```python
from build123d import *

# Parameters (mm, degrees)
CROQUIS1_W                = 220
CROQUIS1_H                = 153
SALIENTE_EXTRUIR1_DEPTH   = 3
CROQUIS2_W                = 160
CROQUIS2_H                = 94
CORTAR_EXTRUIR1_DEPTH     = 4
CROQUIS3_R                = 4.1
CORTAR_EXTRUIR2_DEPTH     = 4
CROQUIS4_R                = 5
SALIENTE_EXTRUIR2_DEPTH   = 7
CROQUIS5_R                = 1.5
CORTAR_EXTRUIR3_DEPTH     = 11
CORTAR_EXTRUIR4_DEPTH     = 3
SIMETR_A2_COPY_1_SKETCH_R = 4.1
SIMETR_A2_COPY_1_DEPTH    = 4
SIMETR_A2_COPY_2_SKETCH_R = 5
SIMETR_A2_COPY_2_DEPTH    = 7
SIMETR_A2_COPY_3_SKETCH_R = 1.5
SIMETR_A2_COPY_3_DEPTH    = 11
SIMETR_A2_COPY_4_DEPTH    = 3
SIMETR_A2_COPY_5_SKETCH_R = 5
SIMETR_A2_COPY_5_DEPTH    = 7
SIMETR_A2_COPY_6_SKETCH_R = 1.5
SIMETR_A2_COPY_6_DEPTH    = 11
SIMETR_A2_COPY_7_DEPTH    = 3


with BuildPart() as part:
    # Croquis1 → Saliente-Extruir1 (new body)
    with BuildSketch(Plane(origin=(0, 0, 0), x_dir=(1, 0, 0), z_dir=(0, 1, 0))):
        Rectangle(CROQUIS1_W, CROQUIS1_H)
    extrude(amount=SALIENTE_EXTRUIR1_DEPTH)

    # Croquis2 → Cortar-Extruir1 (cut, through all)
    with BuildSketch(Plane(origin=(0, 3, 0), x_dir=(1, 0, 0), z_dir=(0, 1, 0))):
        Rectangle(CROQUIS2_W, CROQUIS2_H)
    cortar_extruir1 = extrude(amount=-CORTAR_EXTRUIR1_DEPTH, mode=Mode.SUBTRACT)

    # Croquis3 → Cortar-Extruir2 (cut, through all)
    with BuildSketch(Plane(origin=(0, 3, 0), x_dir=(1, 0, 0), z_dir=(0, 1, 0))):
        with Locations((-100, 61.5)):
            Circle(CROQUIS3_R)
    cortar_extruir2 = extrude(amount=-CORTAR_EXTRUIR2_DEPTH, mode=Mode.SUBTRACT)

    # Croquis4 → Saliente-Extruir2 (add)
    with BuildSketch(Plane(origin=(0, 3, 0), x_dir=(1, 0, 0), z_dir=(0, 1, 0))):
        with Locations((-78.5, 57.5)):
            Circle(CROQUIS4_R)
    saliente_extruir2 = extrude(amount=SALIENTE_EXTRUIR2_DEPTH)

    # Croquis5 → Cortar-Extruir3 (cut, through all)
    with BuildSketch(Plane(origin=(0, 10, 0), x_dir=(1, 0, 0), z_dir=(0, 1, 0))):
        with Locations((-78.5, 57.5)):
            Circle(CROQUIS5_R)
    cortar_extruir3 = extrude(amount=-CORTAR_EXTRUIR3_DEPTH, mode=Mode.SUBTRACT)

    # Croquis6 → Cortar-Extruir4 (cut)
    with BuildSketch(Plane.XZ):
        Polygon((-81.675426481, -57.5), (-80.08771324, -60.25), (-76.91228676, -60.25), (-75.324573519, -57.5), (-76.91228676, -54.75), (-80.08771324, -54.75), align=None)
    cortar_extruir4 = extrude(amount=-CORTAR_EXTRUIR4_DEPTH, mode=Mode.SUBTRACT)

    # Simetría1: Cortar-Extruir2, Saliente-Extruir2, Cortar-Extruir3, Cortar-Extruir4 across plane
    add(cortar_extruir2.mirror(Plane(origin=(0, 0, 0), x_dir=(0, 0, 1), z_dir=(1, 0, 0))), mode=Mode.SUBTRACT)
    add(saliente_extruir2.mirror(Plane(origin=(0, 0, 0), x_dir=(0, 0, 1), z_dir=(1, 0, 0))))
    add(cortar_extruir3.mirror(Plane(origin=(0, 0, 0), x_dir=(0, 0, 1), z_dir=(1, 0, 0))), mode=Mode.SUBTRACT)
    add(cortar_extruir4.mirror(Plane(origin=(0, 0, 0), x_dir=(0, 0, 1), z_dir=(1, 0, 0))), mode=Mode.SUBTRACT)

    # Simetría2: Cortar-Extruir1, Cortar-Extruir2 across plane
    add(cortar_extruir1.mirror(Plane.XY), mode=Mode.SUBTRACT)
    add(cortar_extruir2.mirror(Plane.XY), mode=Mode.SUBTRACT)

    # Simetría2 copy 1 sketch → Simetría2 copy 1 (cut, through all)
    with BuildSketch(Plane(origin=(0, 3, 0), x_dir=(-1, 0, 0), z_dir=(0, 1, 0))):
        with Locations((-100, 61.5)):
            Circle(SIMETR_A2_COPY_1_SKETCH_R)
    extrude(amount=-SIMETR_A2_COPY_1_DEPTH, mode=Mode.SUBTRACT)

    # Simetría2 copy 2 sketch → Simetría2 copy 2 (add)
    with BuildSketch(Plane(origin=(0, 3, 0), x_dir=(-1, 0, 0), z_dir=(0, 1, 0))):
        with Locations((-78.5, 57.5)):
            Circle(SIMETR_A2_COPY_2_SKETCH_R)
    extrude(amount=SIMETR_A2_COPY_2_DEPTH)

    # Simetría2 copy 3 sketch → Simetría2 copy 3 (cut, through all)
    with BuildSketch(Plane(origin=(0, 10, 0), x_dir=(-1, 0, 0), z_dir=(0, 1, 0))):
        with Locations((-78.5, 57.5)):
            Circle(SIMETR_A2_COPY_3_SKETCH_R)
    extrude(amount=-SIMETR_A2_COPY_3_DEPTH, mode=Mode.SUBTRACT)

    # Simetría2 copy 4 sketch → Simetría2 copy 4 (cut)
    with BuildSketch(Plane(origin=(0, 0, 0), x_dir=(-1, 0, 0), z_dir=(0, -1, 0))):
        Polygon((-81.675426481, -57.5), (-80.08771324, -60.25), (-76.91228676, -60.25), (-75.324573519, -57.5), (-76.91228676, -54.75), (-80.08771324, -54.75), align=None)
    extrude(amount=-SIMETR_A2_COPY_4_DEPTH, mode=Mode.SUBTRACT)

    # Simetría2 copy 5 sketch → Simetría2 copy 5 (add)
    with BuildSketch(Plane(origin=(0, 3, 0), x_dir=(1, 0, 0), z_dir=(0, 1, 0))):
        with Locations((-78.5, -57.5)):
            Circle(SIMETR_A2_COPY_5_SKETCH_R)
    extrude(amount=SIMETR_A2_COPY_5_DEPTH)

    # Simetría2 copy 6 sketch → Simetría2 copy 6 (cut, through all)
    with BuildSketch(Plane(origin=(0, 10, 0), x_dir=(1, 0, 0), z_dir=(0, 1, 0))):
        with Locations((-78.5, -57.5)):
            Circle(SIMETR_A2_COPY_6_SKETCH_R)
    extrude(amount=-SIMETR_A2_COPY_6_DEPTH, mode=Mode.SUBTRACT)

    # Simetría2 copy 7 sketch → Simetría2 copy 7 (cut)
    with BuildSketch(Plane.XZ):
        Polygon((-81.675426481, 57.5), (-80.08771324, 60.25), (-76.91228676, 60.25), (-75.324573519, 57.5), (-76.91228676, 54.75), (-80.08771324, 54.75), align=None)
    extrude(amount=-SIMETR_A2_COPY_7_DEPTH, mode=Mode.SUBTRACT)


solid = part.part
```
Source: CAD feature listing. Evaluate the final solid. Frame: model axes, mm. A direction names the side the tool comes from. Coordinates: 2 decimals unless noted, no trailing zeros. Write each loop counter-clockwise with the first axis right and the second up, starting at its lowest first coordinate (ties: lowest second). Pieces come first, ordered by that corner, then holes. Notation, with made-up numbers: (7, 41) -> (26, 41) arc R19 ccw to (26, 51) -> close; hole circle Ø10 at (-36.75, 4.25). An arc over 180 degrees is marked (long way). Return JSON: item names as keys, results as strings. Group by question number.
1) Set-up query: faces 1 (the face through (80, 10, 56)), 2 (the face through (77, 3, 56)), 3 (the face through (75.812, 6.451, 61.716)). Return all of +Z, -Z, +X, -X, +Y, -Y with unobstructed straight access to the full face (end or side cutting, diameter ignored); none if empty.
2) Section query A-A, the plane y = 6.5. Return loops of the section in (x, z).
3) Contact query for flat-ended pins moving along their axis: P1, Ø13, axis at x = -100, z = 61.5, coming from the +Y side; P2, Ø2, axis at x = 73, y = 5.5, coming from the +Z side; P3, Ø5, axis at x = -100, z = -61.5, coming from the +Y side; P4, Ø1.6, axis at x = -78.5, z = -58.5, coming from the -Y side. Output: stop coordinate, or through.
4) Section query D-D, the plane x = 20. Return loops of the section in (y, z), plus the area to 3 significant figures.
5) Section query C-C, the plane z = -2. Return loops of the section in (x, y), plus the area to 3 significant figures.
6) Ray query, line 1 along X through (y, z) = (5.25, -57.5); line 2 along Z through (x, y) = (78.5, 7.5); line 3 along X through (y, z) = (1.05, -61.5). Return the intervals inside material, ascending.
7) Section query B-B, the plane x = -100. Return loops of the section in (y, z), plus the area to 3 significant figures.
8) Mould query, pull axis X, two halves, no side actions, for faces 4 (the face through (-2, 0, -52)), 5 (the face through (-75.812, 6.451, 53.284)). Classes: +X half, -X half, draft (parallel to the pull), parting line (faces both ways), or undercut.
From the geometry:
{
 "1": {"face 1": "+Z, -Z, +X, -X, +Y", "face 2": "-Y", "face 3": "+Y"},
 "2": {"outline": "circle Ø10 at (-78.5, -57.5); circle Ø10 at (-78.5, 57.5); circle Ø10 at (78.5, -57.5); circle Ø10 at (78.5, 57.5); hole circle Ø3 at (-78.5, -57.5); hole circle Ø3 at (-78.5, 57.5); hole circle Ø3 at (78.5, -57.5); hole circle Ø3 at (78.5, 57.5)"},
 "3": {"P1": "y = 3", "P2": "z = 59.68", "P3": "through", "P4": "y = 3"},
 "4": {"outline": "(0, -76.5) -> (3, -76.5) -> (3, -47) -> (0, -47) -> close; (0, 47) -> (3, 47) -> (3, 76.5) -> (0, 76.5) -> close", "area": "177 mm²"},
 "5": {"outline": "(-110, 0) -> (-80, 0) -> (-80, 3) -> (-110, 3) -> close; (80, 0) -> (110, 0) -> (110, 3) -> (80, 3) -> close", "area": "180 mm²"},
 "6": {"line 1": "-83.5 to -80, -77 to -73.5, 73.5 to 77, 80 to 83.5", "line 2": "-62.5 to -59, -56 to -52.5, 52.5 to 56, 59 to 62.5", "line 3": "-110 to -104.1, -95.9 to 95.9, 104.1 to 110"},
 "7": {"outline": "(0, -76.5) -> (3, -76.5) -> (3, -65.6) -> (0, -65.6) -> close; (0, -57.4) -> (3, -57.4) -> (3, 57.4) -> (0, 57.4) -> close; (0, 65.6) -> (3, 65.6) -> (3, 76.5) -> (0, 76.5) -> close", "area": "410 mm²"},
 "8": {"face 4": "draft", "face 5": "undercut"}
}
